Can you work these out from the model? Positions are in its coordinate system, mm. Round coordinates to 2 decimals unless told otherwise and drop trailing zeros. Use one line per item in the form item = value. Start each with the question number.
```python
from build123d import *

# Parameters (mm, degrees)
SKETCH_1_W          = 360
SKETCH_1_H          = 360
EXTRUDE_1_DEPTH     = 5
SKETCH_2_R          = 2.1
CUT_EXTRUDE_1_DEPTH = 255.607541129
FILLET_1_R          = 10
CUT_EXTRUDE_2_DEPTH = 255.607541129
SKETCH_4_R          = 1.6
CUT_EXTRUDE_3_DEPTH = 10
FILLET_2_R          = 2


with BuildPart() as part:
    # 草图1 → 凸台-拉伸1 (new body)
    with BuildSketch(Plane(origin=(0, 0, 0), x_dir=(1, 0, 0), z_dir=(0, 1, 0))):
        Rectangle(SKETCH_1_W, SKETCH_1_H)
    extrude(amount=EXTRUDE_1_DEPTH)

    # 草图2 → 切除-拉伸1 (cut, through all)
    with BuildSketch(Plane(origin=(0, 5, 0), x_dir=(1, 0, 0), z_dir=(0, 1, 0))):
        with Locations(Location((0, 0, 0), (0, 0, 270))):
            Circle(SKETCH_2_R)
        with Locations(Location((40, 0, 0), (0, 0, 270))):
            Circle(SKETCH_2_R)
        with Locations(Location((80, 0, 0), (0, 0, 270))):
            Circle(SKETCH_2_R)
        with Locations(Location((120, 0, 0), (0, 0, 270))):
            Circle(SKETCH_2_R)
        with Locations(Location((160, 0, 0), (0, 0, 270))):
            Circle(SKETCH_2_R)
        with Locations(Location((40, 40, 0), (0, 0, 270))):
            Circle(SKETCH_2_R)
        with Locations(Location((80, 40, 0), (0, 0, 270))):
            Circle(SKETCH_2_R)
        with Locations(Location((120, 40, 0), (0, 0, 270))):
            Circle(SKETCH_2_R)
        with Locations(Location((160, 40, 0), (0, 0, 270))):
            Circle(SKETCH_2_R)
        with Locations(Location((40, 80, 0), (0, 0, 270))):
            Circle(SKETCH_2_R)
        with Locations(Location((80, 80, 0), (0, 0, 270))):
            Circle(SKETCH_2_R)
        with Locations(Location((120, 80, 0), (0, 0, 270))):
            Circle(SKETCH_2_R)
        with Locations(Location((160, 80, 0), (0, 0, 270))):
            Circle(SKETCH_2_R)
        with Locations(Location((40, 120, 0), (0, 0, 270))):
            Circle(SKETCH_2_R)
        with Locations(Location((80, 120, 0), (0, 0, 270))):
            Circle(SKETCH_2_R)
        with Locations(Location((120, 120, 0), (0, 0, 270))):
            Circle(SKETCH_2_R)
        with Locations(Location((160, 120, 0), (0, 0, 270))):
            Circle(SKETCH_2_R)
        with Locations(Location((40, 160, 0), (0, 0, 270))):
            Circle(SKETCH_2_R)
        with Locations(Location((80, 160, 0), (0, 0, 270))):
            Circle(SKETCH_2_R)
        with Locations(Location((120, 160, 0), (0, 0, 270))):
            Circle(SKETCH_2_R)
        with Locations(Location((160, 160, 0), (0, 0, 270))):
            Circle(SKETCH_2_R)
        with Locations(Location((0, 40, 0), (0, 0, 270))):
            Circle(SKETCH_2_R)
        with Locations(Location((0, 80, 0), (0, 0, 270))):
            Circle(SKETCH_2_R)
        with Locations(Location((0, 120, 0), (0, 0, 270))):
            Circle(SKETCH_2_R)
        with Locations(Location((0, 160, 0), (0, 0, 270))):
            Circle(SKETCH_2_R)
        with Locations(Location((0, -160, 0), (0, 0, 90))):
            Circle(SKETCH_2_R)
        with Locations(Location((0, -120, 0), (0, 0, 90))):
            Circle(SKETCH_2_R)
        with Locations(Location((0, -80, 0), (0, 0, 90))):
            Circle(SKETCH_2_R)
        with Locations(Location((0, -40, 0), (0, 0, 90))):
            Circle(SKETCH_2_R)
        with Locations(Location((160, -160, 0), (0, 0, 90))):
            Circle(SKETCH_2_R)
        with Locations(Location((120, -160, 0), (0, 0, 90))):
            Circle(SKETCH_2_R)
        with Locations(Location((80, -160, 0), (0, 0, 90))):
            Circle(SKETCH_2_R)
        with Locations(Location((40, -160, 0), (0, 0, 90))):
            Circle(SKETCH_2_R)
        with Locations(Location((160, -120, 0), (0, 0, 90))):
            Circle(SKETCH_2_R)
        with Locations(Location((120, -120, 0), (0, 0, 90))):
            Circle(SKETCH_2_R)
        with Locations(Location((80, -120, 0), (0, 0, 90))):
            Circle(SKETCH_2_R)
        with Locations(Location((40, -120, 0), (0, 0, 90))):
            Circle(SKETCH_2_R)
        with Locations(Location((160, -80, 0), (0, 0, 90))):
            Circle(SKETCH_2_R)
        with Locations(Location((120, -80, 0), (0, 0, 90))):
            Circle(SKETCH_2_R)
        with Locations(Location((80, -80, 0), (0, 0, 90))):
            Circle(SKETCH_2_R)
        with Locations(Location((40, -80, 0), (0, 0, 90))):
            Circle(SKETCH_2_R)
        with Locations(Location((160, -40, 0), (0, 0, 90))):
            Circle(SKETCH_2_R)
        with Locations(Location((120, -40, 0), (0, 0, 90))):
            Circle(SKETCH_2_R)
        with Locations(Location((80, -40, 0), (0, 0, 90))):
            Circle(SKETCH_2_R)
        with Locations(Location((40, -40, 0), (0, 0, 90))):
            Circle(SKETCH_2_R)
        with Locations(Location((-40, -40, 0), (0, 0, 270))):
            Circle(SKETCH_2_R)
        with Locations(Location((-80, -40, 0), (0, 0, 270))):
            Circle(SKETCH_2_R)
        with Locations(Location((-120, -40, 0), (0, 0, 270))):
            Circle(SKETCH_2_R)
        with Locations(Location((-160, -40, 0), (0, 0, 270))):
            Circle(SKETCH_2_R)
        with Locations(Location((-40, -80, 0), (0, 0, 270))):
            Circle(SKETCH_2_R)
        with Locations(Location((-80, -80, 0), (0, 0, 270))):
            Circle(SKETCH_2_R)
        with Locations(Location((-120, -80, 0), (0, 0, 270))):
            Circle(SKETCH_2_R)
        with Locations(Location((-160, -80, 0), (0, 0, 270))):
            Circle(SKETCH_2_R)
        with Locations(Location((-40, -120, 0), (0, 0, 270))):
            Circle(SKETCH_2_R)
        with Locations(Location((-80, -120, 0), (0, 0, 270))):
            Circle(SKETCH_2_R)
        with Locations(Location((-120, -120, 0), (0, 0, 270))):
            Circle(SKETCH_2_R)
        with Locations(Location((-160, -120, 0), (0, 0, 270))):
            Circle(SKETCH_2_R)
        with Locations(Location((-40, -160, 0), (0, 0, 270))):
            Circle(SKETCH_2_R)
        with Locations(Location((-80, -160, 0), (0, 0, 270))):
            Circle(SKETCH_2_R)
        with Locations(Location((-120, -160, 0), (0, 0, 270))):
            Circle(SKETCH_2_R)
        with Locations(Location((-160, -160, 0), (0, 0, 270))):
            Circle(SKETCH_2_R)
        with Locations(Location((-160, 160, 0), (0, 0, 90))):
            Circle(SKETCH_2_R)
        with Locations(Location((-120, 160, 0), (0, 0, 90))):
            Circle(SKETCH_2_R)
        with Locations(Location((-80, 160, 0), (0, 0, 90))):
            Circle(SKETCH_2_R)
        with Locations(Location((-40, 160, 0), (0, 0, 90))):
            Circle(SKETCH_2_R)
        with Locations(Location((-160, 120, 0), (0, 0, 90))):
            Circle(SKETCH_2_R)
        with Locations(Location((-120, 120, 0), (0, 0, 90))):
            Circle(SKETCH_2_R)
        with Locations(Location((-80, 120, 0), (0, 0, 90))):
            Circle(SKETCH_2_R)
        with Locations(Location((-40, 120, 0), (0, 0, 90))):
            Circle(SKETCH_2_R)
        with Locations(Location((-160, 80, 0), (0, 0, 90))):
            Circle(SKETCH_2_R)
        with Locations(Location((-120, 80, 0), (0, 0, 90))):
            Circle(SKETCH_2_R)
        with Locations(Location((-80, 80, 0), (0, 0, 90))):
            Circle(SKETCH_2_R)
        with Locations(Location((-40, 80, 0), (0, 0, 90))):
            Circle(SKETCH_2_R)
        with Locations(Location((-160, 40, 0), (0, 0, 90))):
            Circle(SKETCH_2_R)
        with Locations(Location((-120, 40, 0), (0, 0, 90))):
            Circle(SKETCH_2_R)
        with Locations(Location((-80, 40, 0), (0, 0, 90))):
            Circle(SKETCH_2_R)
        with Locations(Location((-40, 40, 0), (0, 0, 90))):
            Circle(SKETCH_2_R)
        with Locations(Location((-160, 0, 0), (0, 0, 90))):
            Circle(SKETCH_2_R)
        with Locations(Location((-120, 0, 0), (0, 0, 90))):
            Circle(SKETCH_2_R)
        with Locations(Location((-80, 0, 0), (0, 0, 90))):
            Circle(SKETCH_2_R)
        with Locations(Location((-40, 0, 0), (0, 0, 90))):
            Circle(SKETCH_2_R)
    extrude(amount=-CUT_EXTRUDE_1_DEPTH, mode=Mode.SUBTRACT)

    # 圆角1
    fillet_1_edges = [part.edges().sort_by_distance(p)[0] for p in [
        (180, 2.5, 180),
        (-180, 2.5, 180),
        (-180, 2.5, -180),
        (180, 2.5, -180),
    ]]
    fillet(fillet_1_edges, radius=FILLET_1_R)

    # 草图3 → 切除-拉伸2 (cut, through all)
    with BuildSketch(Plane(origin=(0, 5, 0), x_dir=(1, 0, 0), z_dir=(0, 1, 0))):
        Polygon((5, -180), (5, -170), (20, -170), (20, -150), (-20, -150), (-20, -170), (-5, -170), (-5, -180), align=None)
    extrude(amount=-CUT_EXTRUDE_2_DEPTH, mode=Mode.SUBTRACT)

    # 草图4 → 切除-拉伸3 (cut)
    with BuildSketch(Plane(origin=(0, 5, 0), x_dir=(1, 0, 0), z_dir=(0, 1, 0))):
        with Locations(Location((98, 98, 0), (0, 0, 270))):
            Circle(SKETCH_4_R)
        with Locations(Location((98, -98, 0), (0, 0, 270))):
            Circle(SKETCH_4_R)
        with Locations(Location((-98, -98, 0), (0, 0, 270))):
            Circle(SKETCH_4_R)
        with Locations(Location((-98, 98, 0), (0, 0, 270))):
            Circle(SKETCH_4_R)
        with Locations(Location((98, 0, 0), (0, 0, 270))):
            Circle(SKETCH_4_R)
        with Locations(Location((-98, 0, 0), (0, 0, 270))):
            Circle(SKETCH_4_R)
        with Locations(Location((0, 98, 0), (0, 0, 270))):
            Circle(SKETCH_4_R)
        with Locations(Location((0, -98, 0), (0, 0, 270))):
            Circle(SKETCH_4_R)
    extrude(amount=-CUT_EXTRUDE_3_DEPTH, mode=Mode.SUBTRACT)

    # 圆角2
    fillet_2_edges = [part.edges().sort_by_distance(p)[0] for p in [
        (-5, 2.5, 180),
        (-5, 2.5, 170),
        (-20, 2.5, 170),
        (-20, 2.5, 150),
        (20, 2.5, 150),
        (20, 2.5, 170),
        (5, 2.5, 170),
        (5, 2.5, 180),
    ]]
    fillet(fillet_2_edges, radius=FILLET_2_R)


solid = part.part
```
1. If we section it at A-A (y = 1.2): State how many separate pieces and enclosed holes the cut face has, and give its area (3 significant figures).
2. Please list where these lines run through material, in increasing order: line 1 along Z through (x, y) = (-98, 3.45); line 2 along X through (y, z) = (0.45, 157.5); line 3 along Z through (x, y) = (17.5, 3.75).
3. If we mould it in two halves opening along Z, with no side actions, what happens to faces 1 (the face through (176.99, 2.54, 177.15)), 2 (the face through (-3, 5, -3)), 3 (the face through (-177.15, 2.54, -176.99))? For each: pulls with the +Z half, pulls with the -Z half, needs draft (parallel to the pull), parting line crosses it, or undercut.
Model answer:
q1.separate_pieces = 1
q1.enclosed_holes = 88
q1.area = 127,000 mm2
q2.line_1 = -180 to -99.6, -96.4 to -1.6, 1.6 to 96.4, 99.6 to 180
q2.line_2 = -180 to -20, 20 to 180
q2.line_3 = -180 to 150, 170 to 180
q3.face_1 = pulls with the +Z half
q3.face_2 = needs draft
q3.face_3 = pulls with the -Z half
